Can you work these out from the model? Positions are in its coordinate system, mm. Face numbers are marked on the shaded views. A direction names the side the tool comes from. Round coordinates to 2 decimals unless told otherwise and drop trailing zeros. Write each loop counter-clockwise with the first axis right and the second up, starting at its lowest first coordinate (ties: lowest second). Pieces come first, ordered by that corner, then holes. Notation, with made-up numbers: (89.25, 19) - (116.25, 19) arc R22 cw to (116.25, 57) - close; hole circle Ø11 at (21.5, 9.25). An arc over 180 degrees is marked (long way). One line per item, written item: value. Start each with the question number.
(1) I'm going to push flat-ended pins straight in: pin 1 Ø2.5 at (x, z) = (-22.5, -3.5) entering from +Y (3 decimals); pin 2 Ø4 at (y, z) = (6.5, -2.5) entering from +X (3 decimals); pin 3 Ø8.5 at (x, z) = (-9.5, -5) entering from -Y (3 decimals). Where does each tip first touch, or does it pass through?
(2) If I drill on L1, parallel to Y at x = -22.5, z = 16.5; L2, parallel to X at y = 11, z = 16; L3, parallel to Z at x = 18, y = 2, over which ranges is the centre line in solid material (lowest first)? Write a range as from..to.
(3) I want a section at B-B on y = 11. List the corners of the cut face in (x, z) for me (3 decimals), plus the area to 3 significant figures.
(4) I want a section at A-A on z = 21. List the corners of the cut face in (x, y) for me, plus the area to 3 significant figures.
(5) On a 3-axis mill with a long thin cutter (end or side, diameter ignored), from which of +Z, -Z, +X, -X, +Y, -Y can I reach the whole of each face in a straight line? I mean the marked faces 1 and 2. Say none if no direction works.
(6) Thinking about a two-plate mould opening in Y: for the marked faces 3, 4 and 5, which applies, +Y half, -Y half, draft (parallel to the pull), parting line (faces both ways), or undercut?
(7) I want a section at D-D on z = -5. List the corners of the cut face in (x, y) for me (3 decimals), plus the area to 3 significant figures.
(8) I want a section at C-C on x = 13. List the corners of the cut face in (y, z) for me (3 decimals).
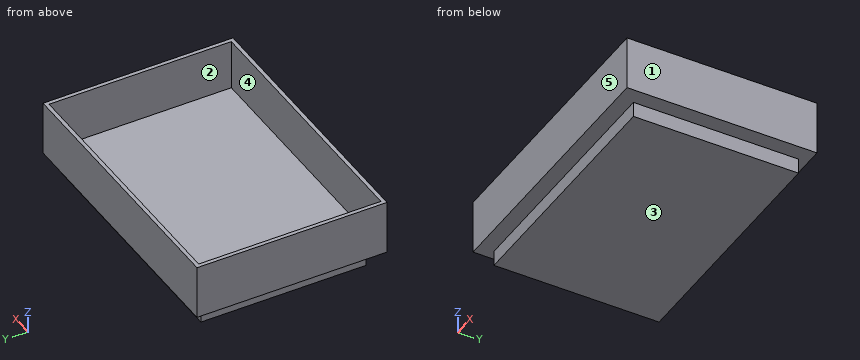
Autodesk Fusion 360 part; units mm, degrees
sketch "Sketch1" plane through (0, 0, 0) normal (0, 0, 1) x (1, 0, 0)
  line L0 (63.375, 42.565) -> (-63.375, 42.565)
  line L1 (-63.375, 42.565) -> (-63.375, -42.565)
  line L2 (-63.375, -42.565) -> (63.375, -42.565)
  line L3 (63.375, -42.565) -> (63.375, 42.565)
  line L4 (63.375, 42.565) -> (-63.375, -42.565) construction
  line L5 (-63.375, 42.565) -> (63.375, -42.565) construction
  line L6 (-68.375, 47.565) -> (68.375, 47.565)
  line L7 (68.375, 47.565) -> (68.375, -47.565)
  line L8 (68.375, -47.565) -> (-68.375, -47.565)
  line L9 (-68.375, -47.565) -> (-68.375, 47.565)
  line L10 (-68.375, 47.565) -> (68.375, -47.565) construction
  line L11 (68.375, 47.565) -> (-68.375, -47.565) construction
  line L12 (71.5, 47.565) -> (68.5, 47.565)
  line L13 (68.5, 47.565) -> (68.5, -47.565)
  line L14 (68.5, -47.565) -> (71.5, -47.565)
  line L15 (71.5, -47.565) -> (71.5, 47.565)
  line L16 (71.5, 47.565) -> (68.5, -47.565) construction
  line L17 (68.5, 47.565) -> (71.5, -47.565) construction
  line L18 (71.4437, -50.4298) -> (-68.3063, -50.4298)
  line L19 (-68.3063, -50.4298) -> (-68.3063, -47.4298)
  line L20 (-68.3063, -47.4298) -> (71.4437, -47.4298)
  line L21 (71.4437, -47.4298) -> (71.4437, -50.4298)
  line L22 (71.4437, -50.4298) -> (-68.3063, -47.4298) construction
  line L23 (-68.3063, -50.4298) -> (71.4437, -47.4298) construction
  point P0 (70, 0)
  point P1 (1.5687, -48.9298)
  dimension "d1" = 126.75
  dimension "d2" = 85.13
  dimension "d3" = 136.75
  dimension "d4" = 95.13
  dimension "d5" = 3
  dimension "d6" = 139.75
  dimension "d7" = 3
sketch "Sketch2" plane through (0, 0, 0) normal (0, 0, 1) x (1, 0, 0)
sketch "Sketch3" plane through (0, 0, 0) normal (0, 0, 1) x (1, 0, 0)
  line L0 (71.4782, -50.4736) -> (-68.4999, -50.4736)
  line L1 (-68.4999, -50.4736) -> (-68.4999, 47.4954)
  line L2 (-68.4999, 47.4954) -> (71.4782, 47.4954)
  line L3 (71.4782, 47.4954) -> (71.4782, -50.4736)
extrude "Extrude1" add sketch "Sketch3" along normal blind 28
shell "Shell1" thickness 2 removed faces 1 at (-21.8406, -17.8173, 28)
extrude "Extrude2" add sketch "Sketch1" against normal blind 3 contours L0 L1 L2 L3
extrude "Extrude3" add 1 faces at (-21.125, -14.1883, -3) along direction (0, 0, -1) blind 4.9
Established:
1. pin 1: y = 42.565
1. pin 2: x = 63.375
1. pin 3: y = -42.565
2. L1: -50.47..-48.47, 45.5..47.5
2. L2: -68.5..-66.5, 69.48..71.48
2. L3: -7.9..2
3. outline: (-68.5, 0) - (-63.375, 0) - (-63.375, -7.9) - (63.375, -7.9) - (63.375, 0) - (71.478, 0) - (71.478, 28) - (69.478, 28) - (69.478, 2) - (-66.5, 2) - (-66.5, 28) - (-68.5, 28) - close
3. area: 1,390 mm2
4. outline: (-68.5, -50.47) - (71.48, -50.47) - (71.48, 47.5) - (-68.5, 47.5) - close; hole (-66.5, -48.47) - (69.48, -48.47) - (69.48, 45.5) - (-66.5, 45.5) - close
4. area: 936 mm2
5. face 1: +Z, -Z, +X, +Y, -Y
5. face 2: +Z
6. face 3: draft
6. face 4: undercut
6. face 5: -Y half
7. outline: (-63.375, -42.565) - (63.375, -42.565) - (63.375, 42.565) - (-63.375, 42.565) - close
7. area: 10,800 mm2
8. outline: (-50.474, 0) - (-42.565, 0) - (-42.565, -7.9) - (42.565, -7.9) - (42.565, 0) - (47.495, 0) - (47.495, 28) - (45.495, 28) - (45.495, 2) - (-48.474, 2) - (-48.474, 28) - (-50.474, 28) - close
